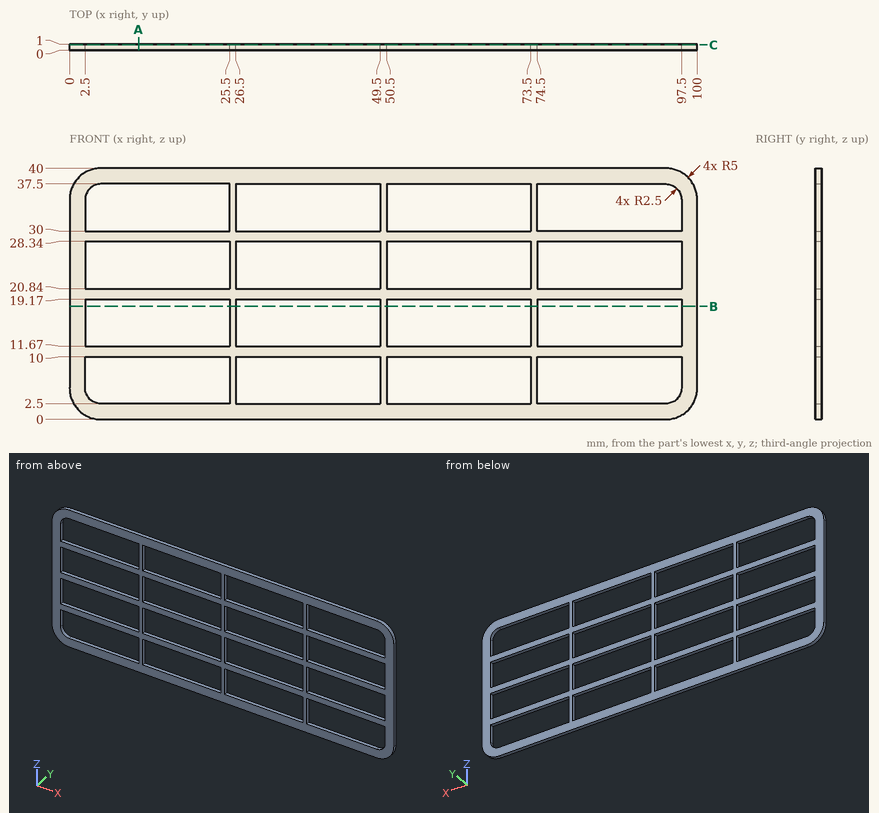
Could you check a few things on this drawing? It's one solid part, dimensions in mm from its lowest x, y, z. Round coordinates to 2 decimals unless told otherwise and drop trailing zeros. Order: outer loops, then holes, each group sorted by start corner. A loop starts at its lowest first (then second) coordinate and runs counter-clockwise, first axis right, second up. Notation, with made-up numbers: M 32.25,-38.75 L 77.25,-38.75 A10 ccw 77.25,-28.75 Z; hole C 68,39.25 d1. An arc over 180 degrees is marked long. Return JSON: item names as keys, results as strings. Group by question number.
1. If we section it at A-A on x = 11: List the corners of the cut face in (y, z) for me.
2. If we section it at C-C on y = 0.85: State how many separate pieces and enclosed holes the cut face has, then the cut area to 3 significant figures.
3. If we section it at B-B on z = 18: List the corners of the cut face in (x, y) for me, then the cut area to 3 significant figures.
4. Please list where these lines run through material, in increasing order: probe 1 along X at (y, z) = (0.25, 22); probe 2 along Z at (x, y) = (20, 0.95); probe 3 along X at (y, z) = (0.65, 36).
Reply:
{
 "1": {"outline": "M 0,0 L 1,0 L 1,2.5 L 0,2.5 Z; M 0,10 L 1,10 L 1,11.67 L 0,11.67 Z; M 0,19.17 L 1,19.17 L 1,20.84 L 0,20.84 Z; M 0,28.34 L 1,28.34 L 1,30 L 0,30 Z; M 0,37.5 L 1,37.5 L 1,40 L 0,40 Z"},
 "2": {"separate pieces": "1", "enclosed holes": "16", "area": "1,220 mm^2"},
 "3": {"outline": "M 0,0 L 2.5,0 L 2.5,1 L 0,1 Z; M 25.5,0 L 26.5,0 L 26.5,1 L 25.5,1 Z; M 49.5,0 L 50.5,0 L 50.5,1 L 49.5,1 Z; M 73.5,0 L 74.5,0 L 74.5,1 L 73.5,1 Z; M 97.5,0 L 100,0 L 100,1 L 97.5,1 Z", "area": "8.00 mm^2"},
 "4": {"probe 1": "0 to 2.5, 25.5 to 26.5, 49.5 to 50.5, 73.5 to 74.5, 97.5 to 100", "probe 2": "0 to 2.5, 10 to 11.67, 19.17 to 20.84, 28.34 to 30, 37.5 to 40", "probe 3": "0.1 to 2.71, 25.5 to 26.5, 49.5 to 50.5, 73.5 to 74.5, 97.29 to 99.9"}
}
